Geometry check sheet. Reference: the model listing, model coordinates, mm. Face numbers are marked on the shaded views. A direction names the side the tool comes from. Round coordinates to 2 decimals unless told otherwise and drop trailing zeros. Loops run counter-clockwise (first coordinate to the right, second up) from the corner with the lowest first, then second, coordinate; pieces in that order, holes last. Notation, with made-up numbers: (-10.5, -32) -> (46.5, -32) arc R20 ccw to (46.5, -21) -> close; hole circle Ø1 at (33, -3.75). An arc over 180 degrees is marked (long way). Use a Markdown table: item, result. Add a question column.
Q1. Sectioned sample at D-D, the plane z = 21. Enter the section's corners in (x, y).
Q2. Sectioned sample at B-B, the plane z = 12.5. Enter the section's corners in (x, y), then the cut area to 3 significant figures.
Q3. Material ranges on L1, parallel to Z at x = 0, y = 5.5; L2, parallel to Z at x = -8.5, y = 5; L3, parallel to Y at x = -3, z = 21, recorded low to high.
Q4. Sectioned sample at A-A, the plane x = 0. Give the number of separate pieces and of enclosed holes in the cut face, then the cut area to 3 significant figures.
Q5. Gauge pin test, flat ends, axial feed: P1, Ø5.5, axis at x = 1, z = 13, coming from the +Y side; P2, Ø5, axis at y = 7.5, z = 6.5, coming from the -X side; P3, Ø8, axis at y = 6.5, z = 17, coming from the -X side. Record the tip position at first contact, or that the pin passes through.
Q6. Set-up check for the marked faces 1 and 2: record each of +Z, -Z, +X, -X, +Y, -Y from which the full face is reachable in a straight line by a thin tool's end or side.
Q7. Release check for a two-part mould opening along Z. For the marked faces 3, 4, 5 and 6 record: released by +Z, released by -Z, zero draft, split by the parting line, or undercut.
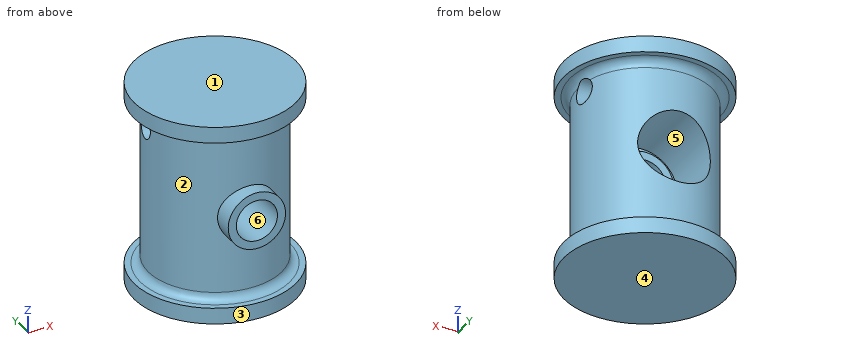
```python
from build123d import *

# Parameters (mm, degrees)
SKIZZE1_R                            = 10
AUFSATZ_LINEAR_AUSTRAGEN1_DEPTH      = 2
SKIZZE2_R                            = 8.25
AUFSATZ_LINEAR_AUSTRAGEN2_DEPTH      = 21
SKIZZE3_R                            = 10
AUFSATZ_LINEAR_AUSTRAGEN3_DEPTH      = 2
VERRUNDUNG1_R                        = 1
SCHNITT_LINEAR_AUSTRAGEN1_DEPTH      = 14
SCHNITT_LINEAR_AUSTRAGEN1_DEPTH_BACK = 14
SKIZZE4_R                            = 1.5
SCHNITT_LINEAR_AUSTRAGEN2_DEPTH      = 14
SCHNITT_LINEAR_AUSTRAGEN2_DEPTH_BACK = 1
SKIZZE5_R                            = 4.5
SKIZZE6_R                            = 2.55
SCHNITT_LINEAR_AUSTRAGEN3_DEPTH      = 14
SKIZZE7_R                            = 3.55
SKIZZE7_R_2                          = 2.55
AUFSATZ_LINEAR_AUSTRAGEN4_DEPTH      = 10


with BuildPart() as part:
    # Skizze1 → Aufsatz-Linear austragen1 (new body)
    with BuildSketch(Plane.XY):
        Circle(SKIZZE1_R)
    extrude(amount=AUFSATZ_LINEAR_AUSTRAGEN1_DEPTH)

    # Skizze2 → Aufsatz-Linear austragen2 (add)
    with BuildSketch(Plane.XY.offset(2)):
        with Locations(Location((0, 0, 0), (0, 0, 180))):
            Circle(SKIZZE2_R)
    extrude(amount=AUFSATZ_LINEAR_AUSTRAGEN2_DEPTH)

    # Skizze3 → Aufsatz-Linear austragen3 (add)
    with BuildSketch(Plane.XY.offset(23)):
        Circle(SKIZZE3_R)
    extrude(amount=AUFSATZ_LINEAR_AUSTRAGEN3_DEPTH)

    # Verrundung1
    verrundung1_edges = [part.edges().sort_by_distance(p)[0] for p in [
        (8.25, 0, 2),
        (8.25, 0, 23),
    ]]
    fillet(verrundung1_edges, radius=VERRUNDUNG1_R)

    # Skizze4 → Schnitt-Linear austragen1 (cut, two sides: drawn at the far end of the back side and taken through both)
    with BuildSketch(Plane.ZY.offset(-SCHNITT_LINEAR_AUSTRAGEN1_DEPTH_BACK)):
        with Locations(Location((21, 1.05, 0), (0, 0, 311.810314887))):
            Circle(SKIZZE4_R)
    extrude(amount=SCHNITT_LINEAR_AUSTRAGEN1_DEPTH + SCHNITT_LINEAR_AUSTRAGEN1_DEPTH_BACK, mode=Mode.SUBTRACT)

    # Skizze5 → Schnitt-Linear austragen2 (cut, two sides: drawn at the far end of the back side and taken through both)
    with BuildSketch(Plane(origin=(0, 0, 0), x_dir=(1, 0, 0), z_dir=(0, 1, 0)).offset(-SCHNITT_LINEAR_AUSTRAGEN2_DEPTH_BACK)):
        with Locations(Location((0, -12.5, 0), (0, 0, 270))):
            Circle(SKIZZE5_R)
    extrude(amount=SCHNITT_LINEAR_AUSTRAGEN2_DEPTH + SCHNITT_LINEAR_AUSTRAGEN2_DEPTH_BACK, mode=Mode.SUBTRACT)

    # Skizze6 → Schnitt-Linear austragen3 (cut)
    with BuildSketch(Plane(origin=(0, -1, 0), x_dir=(1, 0, 0), z_dir=(0, 1, 0))):
        with Locations(Location((0, -12.5, 0), (0, 0, 270))):
            Circle(SKIZZE6_R)
    extrude(amount=-SCHNITT_LINEAR_AUSTRAGEN3_DEPTH, mode=Mode.SUBTRACT)

    # Skizze7 → Aufsatz-Linear austragen4 (add)
    with BuildSketch(Plane(origin=(0, 0, 0), x_dir=(1, 0, 0), z_dir=(0, 1, 0))):
        with Locations(Location((0, -12.5, 0), (0, 0, 270))):
            Circle(SKIZZE7_R)
        with Locations(Location((0, -12.5, 0), (0, 0, 270))):
            Circle(SKIZZE7_R_2, mode=Mode.SUBTRACT)
    extrude(amount=-AUFSATZ_LINEAR_AUSTRAGEN4_DEPTH)


solid = part.part
```
Values:
| question | item | result |
|---|---|---|
| 1 | outline | (-8.24, -0.45) arc R8.25 ccw to (8.24, -0.45) -> close; (-7.85, 2.55) -> (7.85, 2.55) arc R8.25 ccw to start |
| 2 | outline | (-4.5, -1) -> (-4.5, 6.91) arc R8.25 ccw to (-3.55, -7.45) -> (-3.55, -10) -> (-2.55, -10) -> (-2.55, 0) -> (-3.55, 0) -> (-3.55, -1) -> close; (2.55, -10) -> (3.55, -10) -> (3.55, -7.45) arc R8.25 ccw to (4.5, 6.91) -> (4.5, -1) -> (3.55, -1) -> (3.55, 0) -> (2.55, 0) -> close |
| 2 | area | 105 mm^2 |
| 3 | L1 | 0 to 8, 17 to 25 |
| 3 | L2 | 0 to 2, 23 to 25 |
| 3 | L3 | -7.69 to -0.45, 2.55 to 7.69 |
| 4 | separate pieces | 2 |
| 4 | enclosed holes | 1 |
| 4 | area | 306 mm^2 |
| 5 | P1 | y = 0 |
| 5 | P2 | x = -6.56 |
| 5 | P3 | x = -7.86 |
| 6 | face 1 | +Z, +X, -X, +Y, -Y |
| 6 | face 2 | none |
| 7 | face 3 | zero draft |
| 7 | face 4 | released by -Z |
| 7 | face 5 | undercut |
| 7 | face 6 | undercut |
